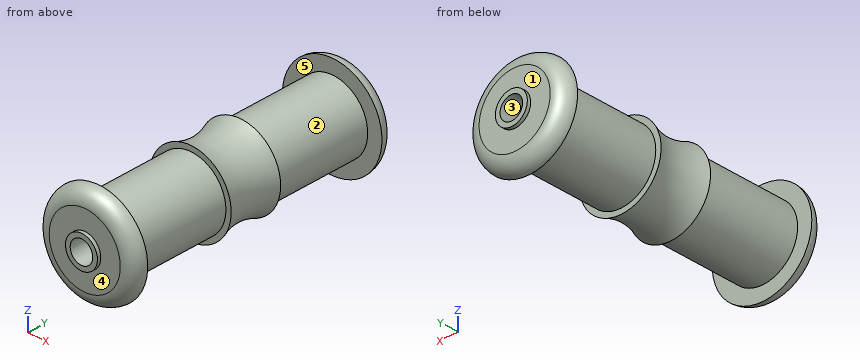
Autodesk Inventor part; units mm, degrees
ref_plane "YZ Plane" through (0, 0, 0) normal (1, 0, 0) x (0, 1, 0)
ref_plane "XZ Plane" through (0, 0, 0) normal (0, 1, 0) x (-1, 0, 0)
ref_plane "XY Plane" through (0, 0, 0) normal (0, 0, 1) x (1, 0, 0)
sketch "Sketch1" plane through (0, 0, 0) normal (0, 1, 0) x (-1, 0, 0)
  circle A0 centre (0, 0) radius 1.5875
  circle A1 centre (0, 0) radius 2.25
  circle A2 centre (0, 0) radius 7
  circle A3 centre (0, 0) radius 5
  circle A4 centre (0, 0) radius 5.75
  dimension "d0" = 3.175
  dimension "d1" = 4.5
  dimension "d2" = 14
  dimension "d3" = 10
  dimension "d4" = 11.5
extrude "Extrusion1" add sketch "Sketch1" against normal blind 0.5 contours A1
extrude "Extrusion2" add sketch "Sketch1" along normal blind 2 contours A1 | A2 | A3 | A4
extrude "Extrusion3" add sketch "Sketch1" along normal blind 14 from surface at 2 contours A1 | A3
extrude "Extrusion4" add sketch "Sketch1" along normal blind 3.75 from surface at 16 contours A1 | A3 | A4
fillet "Fillet1" radius 2 1 edges at (7, 0, 0)
mirror "Mirror1" about plane through (0, 19.75, 0) normal (0, 1, 0)
sketch "Sketch2" plane through (0, 0, 0) normal (1, 0, 0) x (0, 1, 0)
  line L0 (16, -5.75) -> (23.5, -5.75)
  line L1 (16, 5.75) -> (16, -5.75)
  arc A0 (23.5, -5.75) -> (16, -5.75) centre (19.75, -14.75) ccw
  line L2 (0, 0) -> (10, 0) construction
  point P0 (19.75, -5.75)
  point P1 (19.75, -5)
  dimension "d14" = 0.75
  dimension "d15" = 10
revolve "Revolution1" cut sketch "Sketch2" angle 360 about axis through (0, 0, 0) along (0, 1, 0)
properties part number "Dribbler Roller Seperator"
Can you work these out from the model? Positions are in its coordinate system, mm. Face numbers are marked on the shaded views. A direction names the side the tool comes from. Give positions to 0.01 mm unless a question says otherwise; leave off trailing zeros. Loops run counter-clockwise (first coordinate to the right, second up) from the corner with the lowest first, then second, coordinate; pieces in that order, holes last. Notation, with made-up numbers: (43, 63.5) - (98, 63.5) arc R32 ccw to (98, 90.5) - close; hole circle Ø8 at (37.5, 15). An arc over 180 degrees is marked (long way). Return JSON: item names as keys, results as strings.
1. I want a section at A-A on y = 14.5. Please give me the cut outline in (x, z) (1 decimal), and give its area (3 significant figures).
Output values:
{"outline": "circle Ø10 at (0, 0); hole circle Ø3.2 at (0, 0)", "area": "70.6 mm²"}
2. I'm going to push flat-ended pins straight in: pin 1 Ø1.5 at (x, z) = (-4.5, 0.5) entering from -Y; pin 2 Ø4 at (x, y) = (1.5, 34.5) entering from +Z; pin 3 Ø8 at (y, z) = (9, 4.5) entering from -X. Where does each tip first touch, or does it pass through?
Output values:
{"pin 1": "stops at y = 0", "pin 2": "stops at z = 5", "pin 3": "stops at x = -4.97"}
3. We'd pull the mould along Y, two halves only. Please class the marked faces 3, 4 and 5: +Y half, -Y half, draft (parallel to the pull), parting line (faces both ways), or undercut.
Output values:
{"face 3": "draft", "face 4": "-Y half", "face 5": "undercut"}
4. For the marked faces 1 and 2, which set-ups out of +Z, -Z, +X, -X, +Y, -Y let a thin tool reach every point of the face, with its end or its side?
Output values:
{"face 1": "+Y", "face 2": "none"}
5. If I drill on line 1 (Z direction, x = 0, y = 13.5); line 2 (Y direction, x = 3.5, z = 2); line 3 (Y direction, x = 4.5, z = 5), over which ranges is the centre line in solid material (lowest first)?
Output values:
{"line 1": "z = -5 to -1.59, 1.59 to 5", "line 2": "y = 0 to 39.5", "line 3": "y = 0.99 to 2, 37.5 to 38.51"}
